```python
from build123d import *

# Parameters (mm, degrees)
SKETCH1_R           = 0.7
SKETCH1_R_2         = 1.25
BOSS_EXTRUDE1_DEPTH = 1.6
SKETCH2_R           = 3.792840445
SKETCH2_R_2         = 2.43
BOSS_EXTRUDE2_DEPTH = 2.5


with BuildPart() as part:
    # Sketch1 → Boss-Extrude1 (new body)
    with BuildSketch(Plane(origin=(0, 0, 0), x_dir=(1, 0, 0), z_dir=(0, 1, 0))):
        with BuildLine():
            Line((-10.84721718, -1.650301895), (-2.681943198, -2.681943198))
            Line((-2.681943198, -2.681943198), (-1.650301895, -10.84721718))
            ThreePointArc((-1.650301895, -10.84721718), (0, -12.5), (1.650301895, -10.84721718))
            Line((1.650301895, -10.84721718), (2.681943198, -2.681943198))
            Line((2.681943198, -2.681943198), (10.84721718, -1.650301895))
            ThreePointArc((10.84721718, -1.650301895), (12.5, 0), (10.84721718, 1.650301895))
            Line((10.84721718, 1.650301895), (2.681943198, 2.681943198))
            Line((2.681943198, 2.681943198), (1.650301895, 10.84721718))
            ThreePointArc((1.650301895, 10.84721718), (0, 12.5), (-1.650301895, 10.84721718))
            Line((-1.650301895, 10.84721718), (-2.681943198, 2.681943198))
            Line((-2.681943198, 2.681943198), (-10.84721718, 1.650301895))
            ThreePointArc((-10.84721718, 1.650301895), (-12.5, 0), (-10.84721718, -1.650301895))
        make_face()
        with Locations(Location((0, 4.849696243, 0), (0, 0, 270))):
            Circle(SKETCH1_R, mode=Mode.SUBTRACT)
        with Locations(Location((0, 7.849696243, 0), (0, 0, 270))):
            Circle(SKETCH1_R, mode=Mode.SUBTRACT)
        with Locations(Location((0, 10.849696243, 0), (0, 0, 270))):
            Circle(SKETCH1_R, mode=Mode.SUBTRACT)
        with Locations(Location((0, -4.849696243, 0), (0, 0, 90))):
            Circle(SKETCH1_R, mode=Mode.SUBTRACT)
        with Locations(Location((0, -7.849696243, 0), (0, 0, 90))):
            Circle(SKETCH1_R, mode=Mode.SUBTRACT)
        with Locations(Location((0, -10.849696243, 0), (0, 0, 90))):
            Circle(SKETCH1_R, mode=Mode.SUBTRACT)
        with Locations(Location((-10.849696243, 0, 0), (0, 0, 270))):
            Circle(SKETCH1_R, mode=Mode.SUBTRACT)
        with Locations(Location((-7.849696243, 0, 0), (0, 0, 270))):
            Circle(SKETCH1_R, mode=Mode.SUBTRACT)
        with Locations(Location((-4.849696243, 0, 0), (0, 0, 270))):
            Circle(SKETCH1_R, mode=Mode.SUBTRACT)
        with Locations(Location((10.849696243, 0, 0), (0, 0, 90))):
            Circle(SKETCH1_R, mode=Mode.SUBTRACT)
        with Locations(Location((4.849696243, 0, 0), (0, 0, 90))):
            Circle(SKETCH1_R, mode=Mode.SUBTRACT)
        with Locations(Location((7.849696243, 0, 0), (0, 0, 90))):
            Circle(SKETCH1_R, mode=Mode.SUBTRACT)
        with Locations(Location((0, 0, 0), (0, 0, 270))):
            Circle(SKETCH1_R_2, mode=Mode.SUBTRACT)
    extrude(amount=BOSS_EXTRUDE1_DEPTH)

    # Sketch2 → Boss-Extrude2 (add)
    with BuildSketch(Plane.XZ):
        with Locations(Location((0, 0, 0), (0, 0, 45))):
            Circle(SKETCH2_R)
        with Locations(Location((0, 0, 0), (0, 0, 270))):
            Circle(SKETCH2_R_2, mode=Mode.SUBTRACT)
    extrude(amount=BOSS_EXTRUDE2_DEPTH)


solid = part.part
```
The listing builds one solid part. Answer for the finished solid, in the listing's coordinates (mm). A direction names the side the tool comes from. Coordinates: 2 decimals unless noted, no trailing zeros. Loops run counter-clockwise (first coordinate to the right, second up) from the corner with the lowest first, then second, coordinate; pieces in that order, holes last. Notation, with made-up numbers: (63.25, 6) - (118.25, 6) arc R18 ccw to (118.25, 33) - close; hole circle Ø5 at (38.25, 73.5). An arc over 180 degrees is marked (long way). Write item = value, one per line.
1) Section B-B (z = 7.75) is taken. Determine the outline of the cut face in (x, y), plus the area to 3 significant figures.
Responses:
outline = (-2.04, 0) - (-0.69, 0) - (-0.69, 1.6) - (-2.04, 1.6) - close; (0.69, 0) - (2.04, 0) - (2.04, 1.6) - (0.69, 1.6) - close
area = 4.32 mm^2
2) Which of the six approach directions +Z, -Z, +X, -X, +Y, -Y give full straight-line access (tool end or side, diameter ignored) to faces 1 (the face through (-10.26, 0.79, 0.38)), 2 (the face through (-1, 0, -1))?
Responses:
face_1 = +Y, -Y
face_2 = -Y
3) Find the intervals of material crossed by line 1 along X through (y, z) = (-1.5, 1.75); line 2 along Z through (x, y) = (-11.25, 0.9); line 3 along Y through (x, z) = (1.25, 7.5), in increasing order.
Responses:
line_1 = -3.36 to -1.69, 1.69 to 3.36
line_2 = -1.6 to -0.57, 0.57 to 1.6
line_3 = 0 to 1.6
4) This flat-tipped pin is pushed along its axis until it touches: P1, Ø1.8, axis at x = -4.85, z = 0, coming from the -Y side. Where does it stop, or does it pass through?
Responses:
P1 = 0
5) Determine the mould class of faces 3 (the face through (2, -2.5, -2)), 4 (the face through (-2.16, 0.79, -6.82)), 5 (the face through (0, 0.8, 12.5)), 6 (the face through (-1.22, 0.79, -0.27)) for opening direction X: pulls with the +X half, pulls with the -X half, needs draft (parallel to the pull), parting line crosses it, or undercut.
Responses:
face_3 = needs draft
face_4 = pulls with the -X half
face_5 = parting line crosses it
face_6 = undercut
6) Section C-C (z = 0) is taken. Count the separate pieces of the cut face and the enclosed holes in it, plus the area to 3 significant figures.
Responses:
separate_pieces = 8
enclosed_holes = 0
area = 29.4 mm^2
7) Section A-A (x = -5.25) is taken. Determine the outline of the cut face in (y, z).
Responses:
outline = (0, -2.36) - (1.6, -2.36) - (1.6, -0.57) - (0, -0.57) - close; (0, 0.57) - (1.6, 0.57) - (1.6, 2.36) - (0, 2.36) - close
